from build123d import *

# Parameters (mm, degrees)
F0_R     = 17.5
F0_W     = 10
F0_H     = 30
F0_W_2   = 8
F0_H_2   = 15
F1_DEPTH = 15
F2_R     = 4.99999


# Not quite as in the source:
# - a fillet or chamfer is up to 0.001 mm smaller than in the source, because OpenCascade refuses the exact size


with BuildPart() as f1:
    # F0 (on Top) → F1 (new body)
    with BuildSketch(Plane.XY):
        Polygon((-106.1073173197, 0), (0, 0), (0, 25), (-155, 25), (-155, 0), (-145, 0), (-135, 0), (-127, 0), (-120.1073173197, 0), align=None)
        with BuildLine():
            Line((0, 25), (0, 0))
            ThreePointArc((0, 0), (67.6917420766, 12.5), (0, 25))
        make_face()
        with Locations((32.6917420766, 12.5)):
            Circle(F0_R, mode=Mode.SUBTRACT)
        Polygon((-113.1073173197, -15), (-106.1073173197, 0), (-120.1073173197, 0), align=None)
        with Locations((-150, -15)):
            Rectangle(F0_W, F0_H)
        with Locations((-131, -7.5)):
            Rectangle(F0_W_2, F0_H_2)
    extrude(amount=F1_DEPTH)

    # F2 (radius 5 in the source; OpenCascade refuses exactly that, so slightly less here)
    f2_edges = [f1.edges().sort_by_distance(p)[0] for p in [
        (-155, 25, 7.5),
        (-155, -30, 7.5),
        (-150, -30, 15),
        (-145, -15, 0),
        (-140, 0, 0),
        (-135, -7.5, 0),
        (-131, -15, 0),
    ]]
    fillet(f2_edges, radius=F2_R)


solid = f1.part
Build history of the part. All positions in model axes, mm. A direction names the side the tool comes from. Give positions to 0.01 mm unless a question says otherwise; leave off trailing zeros. Order: outer loops, then holes, each group sorted by start corner. A loop starts at its lowest first (then second) coordinate and runs counter-clockwise, first axis right, second up. Notation, with made-up numbers: M 89,-33 L 95,-33 A15 cw 95,-24 Z; hole C 89,-38 d5. An arc over 180 degrees is marked long. Use one line per item in the form item = value.
1) Saw through at C-C (x = -72). Give the cut face in (y, z), plus the area to 3 significant figures.
Calculated:
outline = M 0,0 L 25,0 L 25,15 L 0,15 Z
area = 375 mm2
2) Probe probe 1 along Y at (x, z) = (-126.5, 13.5); probe 2 along X at (y, z) = (-18, 3.25); probe 3 along X at (y, z) = (3.5, 1). List the from-to ranges inside material, lowest first.
Calculated:
probe_1 = 0 to 25
probe_2 = -155 to -145.32, 15.52 to 49.86
probe_3 = -155 to 17.68, 47.7 to 66.51
3) Two-plate mould, pull along X, no slides. Class faces 4 (the face through (-127, -8, 7)), 5 (the face through (-153, 24, 8)), 6 (the face through (-20, 9, 0)): released by +X, released by -X, zero draft, split by the parting line, or undercut.
Calculated:
face_4 = undercut
face_5 = released by -X
face_6 = zero draft
4) Tool access for faces 1 (the face through (-74, 25, 7)), 2 (the face through (-131, -15, 10)), 3 (the face through (-134, -5, 2)): list every direction of +Z, -Z, +X, -X, +Y, -Y with a clear straight run to the whole face (end or side of a thin tool).
Calculated:
face_1 = +Z, -Z, -X, +Y
face_2 = +Z, -Z, -Y
face_3 = -Z, -Y
5) Saw through at B-B (x = 20.5). Give the cut face in (y, z), plus the area to 3 significant figures.
Calculated:
outline = M -20.31,0 L -0.05,0 L -0.05,15 L -20.31,15 Z; M 25.05,0 L 45.31,0 L 45.31,15 L 25.05,15 Z
area = 608 mm2
6) Saw through at A-A (y = 12.5). Give the cut face in (x, z), plus the area to 3 significant figures.
Calculated:
outline = M -155,0 L 15.19,0 L 15.19,15 L -155,15 Z; M 50.19,0 L 67.69,0 L 67.69,15 L 50.19,15 Z
area = 2,820 mm2
7) Drop flat-ended pins along their axis: pin 1 (6 mm diameter, centred on x = -23.5, z = 5.5, fed in from -Y); pin 2 (1.5 mm diameter, centred on x = 32.5, z = 1.5, fed in from -Y); pin 3 (6.5 mm diameter, centred on x = -129.5, z = 10.5, fed in from -Y). Give the stop position or say it passes through.
Calculated:
pin_1 = 0
pin_2 = -22.5
pin_3 = -15
8) Saw through at D-D (y = 41). Give the cut face in (x, z), plus the area to 3 significant figures.
Calculated:
outline = M 12.38,0 L 53.01,0 L 53.01,15 L 12.38,15 Z
area = 609 mm2
